```python
from build123d import *

# Parameters (mm, degrees)
BOSS_EXTRUDE1_DEPTH = 147.955
SKETCH2_W           = 10.4775
SKETCH2_H           = 19.05
CUT_EXTRUDE1_DEPTH  = 162.085115169
SKETCH3_W           = 3.175
SKETCH3_H           = 12.7
CUT_EXTRUDE2_DEPTH  = 162.085115169
SKETCH4_W           = 6.35
SKETCH4_H           = 6.35
SKETCH4_W_2         = 3.175
CUT_EXTRUDE3_DEPTH  = 162.085115169


with BuildPart() as part:
    # Sketch1 → Boss-Extrude1 (new body)
    with BuildSketch(Plane(origin=(0, 0, 0), x_dir=(0, 0, -1), z_dir=(1, 0, 0))):
        with BuildLine():
            Line((1.524, 0), (1.524, -12.7))
            Line((1.524, -12.7), (3.524, -12.7))
            Line((3.524, -12.7), (3.524, 3.175))
            Line((3.524, 3.175), (1.651, 3.175))
            ThreePointArc((1.651, 3.175), (-0.59406403, 4.10493597), (-1.524, 6.35))
            Line((-1.524, 6.35), (-1.524, 63.5))
            Line((-1.524, 63.5), (-3.524, 63.5))
            Line((-3.524, 63.5), (-3.524, -12.7))
            Line((-3.524, -12.7), (-1.524, -12.7))
            Line((-1.524, -12.7), (-1.524, 0))
            Line((-1.524, 0), (1.524, 0))
        make_face()
    extrude(amount=BOSS_EXTRUDE1_DEPTH)

    # Sketch2 → Cut-Extrude1 (cut, through all)
    with BuildSketch(Plane(origin=(0, 0, 1.524), x_dir=(-1, 0, 0), z_dir=(0, 0, -1))):
        with Locations((-142.71625, -3.175)):
            Rectangle(SKETCH2_W, SKETCH2_H)
        with Locations((-5.23875, -3.175)):
            Rectangle(SKETCH2_W, SKETCH2_H)
    extrude(amount=CUT_EXTRUDE1_DEPTH, mode=Mode.SUBTRACT)

    # Sketch3 → Cut-Extrude2 (cut, through all)
    with BuildSketch(Plane(origin=(0, 0, 1.524), x_dir=(-1, 0, 0), z_dir=(0, 0, -1))):
        with Locations((-139.065, -6.35)):
            Rectangle(SKETCH3_W, SKETCH3_H)
        with Locations((-8.89, -6.35)):
            Rectangle(SKETCH3_W, SKETCH3_H)
    extrude(amount=-CUT_EXTRUDE2_DEPTH, mode=Mode.SUBTRACT)

    # Sketch4 → Cut-Extrude3 (cut, through all)
    with BuildSketch(Plane(origin=(0, 0, 1.524), x_dir=(-1, 0, 0), z_dir=(0, 0, -1))):
        with Locations((-140.6525, 38.1)):
            Rectangle(SKETCH4_W, SKETCH4_H)
        with Locations((-139.065, 31.75)):
            Rectangle(SKETCH4_W_2, SKETCH4_H)
        Polygon((-10.4775, 41.275), (-10.4775, 34.925), (-7.3025, 34.925), (-4.1275, 34.925), (-4.1275, 41.275), align=None)
        with Locations((-8.89, 31.75)):
            Rectangle(SKETCH4_W_2, SKETCH4_H)
    extrude(amount=-CUT_EXTRUDE3_DEPTH, mode=Mode.SUBTRACT)


solid = part.part
```
The model under review builds one solid part; all positions refer to its coordinate system, in mm. A direction names the side the tool comes from. Round coordinates to 2 decimals unless told otherwise and drop trailing zeros. Loops run counter-clockwise (first coordinate to the right, second up) from the corner with the lowest first, then second, coordinate; pieces in that order, holes last. Notation, with made-up numbers: (37.5, 42) - (73.5, 42) arc R24 ccw to (73.5, 60) - close; hole circle Ø11 at (58, -20.75). An arc over 180 degrees is marked (long way). Write each question's results on one line, items separated by ' | '. Start each with the question number.
Q1. Take a section at C-C on z = 0. Give the boundary of the cut face in (x, y).
Q2. Take a section at A-A on x = 68.5. Give the boundary of the cut face in (y, z) (3 decimals).
Q3. Take a section at B-B on y = 17. Give the boundary of the cut face in (x, z) (3 decimals), plus the area to 3 significant figures.
Q4. Draft analysis for pull direction Z (two halves, no side actions). For faces 4 (the flat face through (10.478, -3, -2)), 5 (the cylindrical face through (73.09, 4.08, 0.57)), 6 (the flat face through (73, 0, 0)), state which applies: pulls with the +Z half, pulls with the -Z half, needs draft (parallel to the pull), parting line crosses it, or undercut.
Q5. Wall thickness on line 1 along X through (y, z) = (-5, 2.5) (1 decimal); line 2 along Z through (x, y) = (71, -4); line 3 along Z through (x, y) = (79.5, 11): over which ranges is each line inside the solid? List them lowest first. Write a range as [from, to].
Q6. Tool access review of faces 1 (the flat face through (73, -6, -1.524)), 2 (the flat face through (73, 26, 3.524)), 3 (the flat face through (137.478, -3, -2)): name each direction out of +Z, -Z, +X, -X, +Y, -Y from which nothing blocks a thin tool from reaching the whole face with its end or side.
Q7. Insertion check: P1, Ø1.5, axis at x = 58, z = 0, coming from the -Y side; P2, Ø6, axis at x = 80.5, y = 13.5, coming from the -Z side; P3, Ø2.5, axis at y = 1.5, z = -0.5, coming from the +X side. Each pin has a flat end and moves straight along its axis. Give the tip position at first contact, or say it passes through.
Data:
1) outline: (10.48, 0) - (137.48, 0) - (137.48, 3.64) - (10.48, 3.64) - close
2) outline: (-12.7, -3.524) - (3.175, -3.524) - (3.175, -1.651) arc R3.175 cw to (6.35, 1.524) - (63.5, 1.524) - (63.5, 3.524) - (-12.7, 3.524) - (-12.7, 1.524) - (0, 1.524) - (0, -1.524) - (-12.7, -1.524) - close
3) outline: (0, 1.524) - (147.955, 1.524) - (147.955, 3.524) - (0, 3.524) - close | area: 296 mm²
4) face 4: needs draft | face 5: pulls with the -Z half | face 6: undercut
5) line 1: x = [0, 7.3], [10.5, 137.5], [140.7, 148] | line 2: z = [-3.52, -1.52], [1.52, 3.52] | line 3: z = [1.52, 3.52]
6) face 1: +X, -X, -Y | face 2: +Z, +X, -X, +Y, -Y | face 3: -Z, +X, +Y, -Y
7) P1: stops at y = 0 | P2: stops at z = 1.52 | P3: stops at x = 137.48
